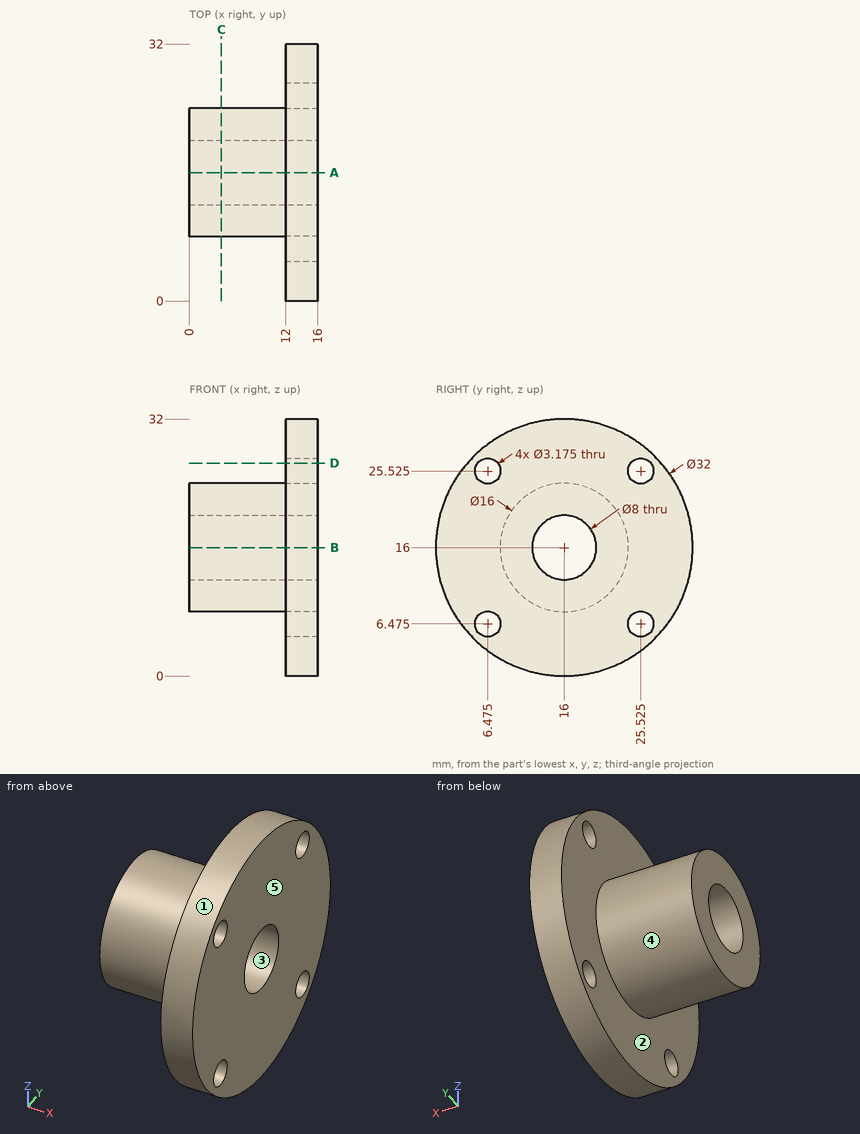
Design review of the part shown in the three views and the two pictorial views. Dimensions are in mm from the part's minimum x, y and z. A direction names the side the tool comes from. Coordinates: 2 decimals unless noted, no trailing zeros. Loops run counter-clockwise (first coordinate to the right, second up) from the corner with the lowest first, then second, coordinate; pieces in that order, holes last.
Q1. The part is to be moulded in two halves that separate along Y. For the marked faces 1, 2 and 3, say which applies: +Y half, -Y half, draft (parallel to the pull), parting line (faces both ways), or undercut.
Reported:
face 1: parting line
face 2: draft
face 3: undercut
Q2. We need section D-D on z = 26.5. State the section outline as (x, y) points.
Reported:
outline: (12, 3.93) - (16, 3.93) - (16, 5.22) - (12, 5.22) - close; (12, 7.73) - (16, 7.73) - (16, 24.27) - (12, 24.27) - close; (12, 26.78) - (16, 26.78) - (16, 28.07) - (12, 28.07) - close
Q3. Tool access review of the marked faces 4 and 5: name each direction out of +Z, -Z, +X, -X, +Y, -Y from which nothing blocks a thin tool from reaching the whole face with its end or side.
Reported:
face 4: -X
face 5: +Z, -Z, +X, +Y, -Y
Q4. We need section A-A on y = 16. State the section outline as (x, z) points.
Reported:
outline: (0, 8) - (12, 8) - (12, 0) - (16, 0) - (16, 12) - (0, 12) - close; (0, 20) - (16, 20) - (16, 32) - (12, 32) - (12, 24) - (0, 24) - close
Q5. For pin 1 (5 mm diameter, centred on y = 25.525, z = 6.475, fed in from -X); pin 2 (1.5 mm diameter, centred on x = 6.5, z = 18.5, fed in from +Y); pin 3 (8 mm diameter, centred on x = 5.5, y = 17, fed in from -Z), all flat-tipped, find the tip position at first contact; note any pin that passes through.
Reported:
pin 1: stops at x = 12
pin 2: stops at y = 23.81
pin 3: stops at z = 8
Q6. We need section C-C on x = 4. State the section outline as (y, z) points, and give its area (3 significant figures).
Reported:
outline: circle Ø16 at (16, 16); hole circle Ø8 at (16, 16)
area: 151 mm2
Q7. To check wall thickness, follow line 1 (Y direction, x = 13.25, z = 26); line 2 (Z direction, x = 2.75, y = 18.5); line 3 (Z direction, x = 12.5, y = 17.5). State the ranges of each line that lie inside material, in increasing order.
Reported:
line 1: y = 3.51 to 4.96, 7.99 to 24.01, 27.04 to 28.49
line 2: z = 8.4 to 12.88, 19.12 to 23.6
line 3: z = 0.07 to 12.29, 19.71 to 31.93
